```python
from build123d import *

# Parameters (mm, degrees)
F3_DEPTH = 25
F5_DEPTH = 1.7
F6_R     = 3
F7_DEPTH = 12.88


with BuildPart() as f1:
    # F0 (on Front) → F1 (revolve)
    with BuildSketch(Plane.XZ):
        Polygon((0, 3.25), (0, 2.85), (1, 3), (3, 3.01), (3, 4), (17, 4), (17, 5), (2, 5), (2, 4.3526792594), align=None)
    revolve(axis=Axis((8.0843353644, 0, 0), (1, 0, 0)))

    # F2 (on face) → F3 (cut)
    with BuildSketch(Plane.YZ.offset(17)):
        Polygon((0, 8.2961460575), (0, 0), (0, -8.2128858194), (10.234137997, -8.383821696), (10.234137997, 8.2961460575), align=None)
    extrude(amount=-F3_DEPTH, mode=Mode.SUBTRACT)

    # F4 (on face) → F5 (join)
    with BuildSketch(Plane(origin=(0, 0, 0), x_dir=(-1, 0, 0), z_dir=(0, 1, 0))):
        with BuildLine():
            Line((-11.0686269666, -4), (-3.1313730334, -4))
            ThreePointArc((-3.1313730334, -4), (-7.1, -2.5), (-11.0686269666, -4))
        make_face()
    extrude(amount=-F5_DEPTH)

    # F6 (on face) → F7 (cut)
    with BuildSketch(Plane.YZ.offset(17)):
        Circle(F6_R)
    extrude(amount=-F7_DEPTH, mode=Mode.SUBTRACT)


solid = f1.part
```
Design review of the part built by this model. Coordinates are the model's own, in mm. A direction names the side the tool comes from. Give positions to 0.01 mm unless a question says otherwise; leave off trailing zeros. Write each loop counter-clockwise with the first axis right and the second up, starting at its lowest first coordinate (ties: lowest second). Pieces come first, ordered by that corner, then holes.
(1) Wall thickness on line 1 along Z through (x, y) = (6, -0.15); line 2 along X through (y, z) = (-3.55, 3.25); line 3 along Z through (x, y) = (6, -2.95): over which ranges is each line inside the solid? List them lowest first.
Checked values:
line 1: z = -5 to -3, 4 to 5
line 2: x = 2 to 17
line 3: z = -4.04 to -2.7, 2.7 to 4.04
(2) Tool access review of faces 1 (the face through (2, -4.55, -0.02)), 2 (the face through (7, -1.7, -3)), 3 (the face through (9, 0, -4)), 4 (the face through (3, -3.4, 0.1)): name each direction out of +Z, -Z, +X, -X, +Y, -Y from which nothing blocks a thin tool from reaching the whole face with its end or side.
Checked values:
face 1: -X, -Y
face 2: +X
face 3: +Z, -Z, +X, -X, +Y
face 4: +Y
(3) Clearance check with flat-ended pins moving along their axes: pin 1 Ø1 at (x, y) = (14.5, -1.5) entering from -Z; pin 2 Ø1.5 at (x, y) = (12.5, -4) entering from +Z. State where each tip first meets the part, or that it passes through.
Checked values:
pin 1: stops at z = -4.9
pin 2: stops at z = 3.8
(4) Add section A-A (x = 11.25). Give the boundary of the cut face in (y, z), and give its area (3 significant figures).
Checked values:
outline: (0, -5) - (0, -4) arc R4 cw to (0, 4) - (0, 5) arc R5 ccw to start
area: 14.1 mm2
(5) Add section B-B (x = 5). Give the boundary of the cut face in (y, z), and give its area (3 significant figures).
Checked values:
outline: (-1.7, -3.62) arc R4 cw to (0, 4) - (0, 5) arc R5 ccw to (0, -5) - (0, -3) arc R3 cw to (-0.84, -2.88) - (-1.7, -2.88) - close
area: 15.8 mm2
(6) Mouldability with a two-part tool opening along Z and no side actions: class faces 5 (the face through (0.4, -2.91, 0.06)), 6 (the face through (17, -4.2, -0.3)), 7 (the face through (0.319, -3.425, 0.075)) as +Z half, -Z half, draft (parallel to the pull), parting line (faces both ways), or undercut.
Checked values:
face 5: undercut
face 6: draft
face 7: parting line
(7) Add section C-C (x = 2.25). Give the boundary of the cut face in (y, z), and give its area (3 significant figures).
Checked values:
outline: (0, -5) - (0, -3.01) arc R3.01 cw to (0, 3.01) - (0, 5) arc R5 ccw to start
area: 25.1 mm2
